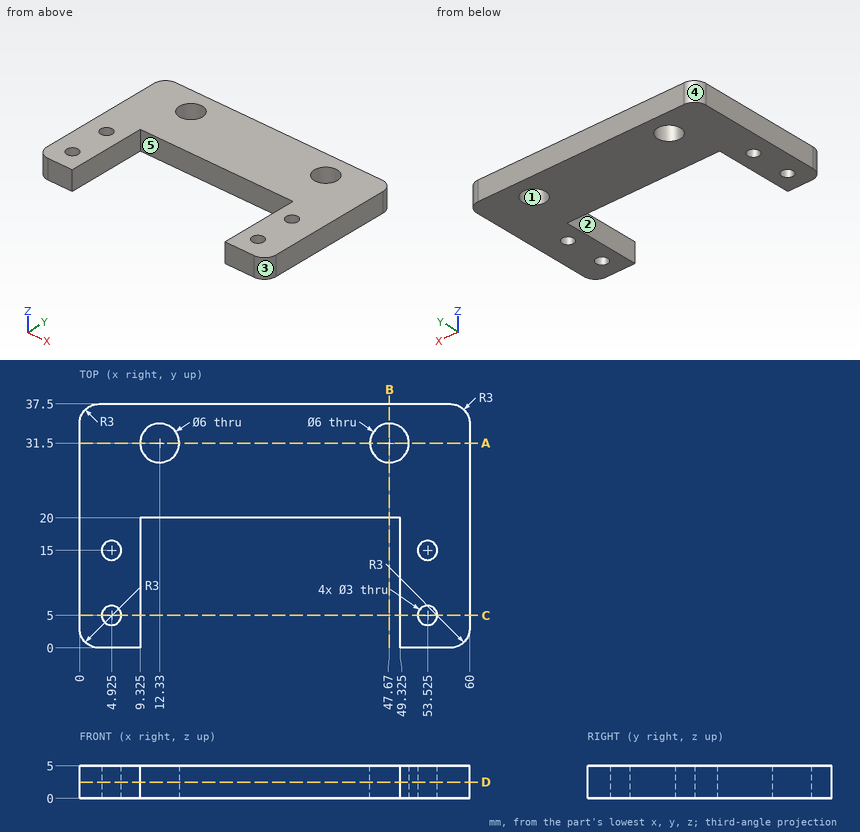
Drawing for the job (mm, zero at the part's lowest x, y, z). A direction names the side the tool comes from. Round coordinates to 2 decimals unless told otherwise and drop trailing zeros. Loops run counter-clockwise (first coordinate to the right, second up) from the corner with the lowest first, then second, coordinate; pieces in that order, holes last. Notation, with made-up numbers: M 68,20.5 L 79,20.5 A8 cw 79,24.5 Z; hole C 48,17 d2. An arc over 180 degrees is marked long. Use a Markdown table: item, result. Add a question column.
(1) Which spindle directions (+Z, -Z, +X, -X, +Y, -Y) get a long thin tool onto all of the face, cutting with end or side? Do the marked faces 4 and 5. Say none if no direction does.
(2) Drill centre lines: line 1 (X direction, y = 7.5, z = 3.8) (3 decimals); line 2 (X direction, y = 30, z = 0.35); line 3 (Y direction, x = 4, z = 2.25). Where is each one in solid material? Low to high.
(3) Cut at A-A (y = 31.5). Give the cut face in (x, z), and give its area (3 significant figures).
(4) Pull direction Y, two halves, no side cores. Call the marked faces 1, 2 and 3: +Y half, -Y half, draft (parallel to the pull), parting line (faces both ways), or undercut.
(5) Cut at D-D (z = 2.5). Give the cut face in (x, y) (3 decimals), and give its area (3 significant figures).
(6) Cut at C-C (y = 5). Give the cut face in (x, z) (3 decimals), and give its area (3 significant figures).
(7) Cut at B-B (x = 47.67). Give the cut face in (y, z), and give its area (3 significant figures).
(8) Flat gauge pins, fed straight in: pin 1 (1.5 mm diameter, centred on x = 32, z = 3, fed in from -Y); pin 2 (2.5 mm diameter, centred on x = 53.525, y = 5, fed in from -Z); pin 3 (3.5 mm diameter, centred on x = 4.925, y = 5, fed in from +Z). Where does each tip first touch, or does it go through?
Geometry says:
| question | item | result |
|---|---|---|
| 1 | face 4 | +Z, -Z, -X, +Y |
| 1 | face 5 | +Z, -Z, -Y |
| 2 | line 1 | x = 0 to 9.325, 49.325 to 60 |
| 2 | line 2 | x = 0 to 9.73, 14.93 to 45.07, 50.27 to 60 |
| 2 | line 3 | y = 0 to 3.82, 6.18 to 13.82, 16.18 to 37.5 |
| 3 | outline | M 0,0 L 9.33,0 L 9.33,5 L 0,5 Z; M 15.33,0 L 44.67,0 L 44.67,5 L 15.33,5 Z; M 50.67,0 L 60,0 L 60,5 L 50.67,5 Z |
| 3 | area | 240 mm² |
| 4 | face 1 | undercut |
| 4 | face 2 | draft |
| 4 | face 3 | -Y half |
| 5 | outline | M 0,3 A3 ccw 3,0 L 9.325,0 L 9.325,20 L 49.325,20 L 49.325,0 L 57,0 A3 ccw 60,3 L 60,34.5 A3 ccw 57,37.5 L 3,37.5 A3 ccw 0,34.5 Z; hole C 4.925,5 d3; hole C 4.925,15 d3; hole C 12.33,31.5 d6; hole C 47.67,31.5 d6; hole C 53.525,5 d3; hole C 53.525,15 d3 |
| 5 | area | 1,360 mm² |
| 6 | outline | M 0,0 L 3.425,0 L 3.425,5 L 0,5 Z; M 6.425,0 L 9.325,0 L 9.325,5 L 6.425,5 Z; M 49.325,0 L 52.025,0 L 52.025,5 L 49.325,5 Z; M 55.025,0 L 60,0 L 60,5 L 55.025,5 Z |
| 6 | area | 70.0 mm² |
| 7 | outline | M 20,0 L 28.5,0 L 28.5,5 L 20,5 Z; M 34.5,0 L 37.5,0 L 37.5,5 L 34.5,5 Z |
| 7 | area | 57.5 mm² |
| 8 | pin 1 | stops at y = 20 |
| 8 | pin 2 | passes through |
| 8 | pin 3 | stops at z = 5 |
